```python
from build123d import *

# Parameters (mm, degrees)
BOSS_EXTRUDE1_DEPTH = 12.7
SKETCH2_R           = 3.175000002
CUT_EXTRUDE1_DEPTH  = 2375.892579794


with BuildPart() as part:
    # Sketch1 → Boss-Extrude1 (new body)
    with BuildSketch(Plane(origin=(-0.000661708, -8255.328766721, 681.010699718), x_dir=(-0.9999999999999969, 7.961414168714261e-08, -6.567661367452003e-09), z_dir=(-7.988457756299225e-08, -0.996614682353027, 0.08221420143970737))):
        Polygon((927.932358973, -1893.28840213), (1306.839320092, -1893.28840213), (1432.35206282, -1316.739819062), (802.419616245, -1316.739819062), align=None)
    extrude(amount=BOSS_EXTRUDE1_DEPTH)

    # Sketch2 → Cut-Extrude1 (cut, through all)
    with BuildSketch(Plane(origin=(-0.000661714, -8255.328766721, 681.010699718), x_dir=(0.9999999999999968, -7.961414422751635e-08, 6.5676468617910225e-09), z_dir=(7.988457890219468e-08, 0.9966146823530272, -0.08221420143970452))):
        with Locations(Location((-1284.956595837, -1854.019614904, 0), (0, 0, 270))):
            Circle(SKETCH2_R)
        with Locations(Location((-949.797461581, -1853.938669103, 0), (0, 0, 270))):
            Circle(SKETCH2_R)
        with Locations(Location((-1387.301054815, -1360.701208825, 0), (0, 0, 270))):
            Circle(SKETCH2_R)
        with Locations(Location((-847.47062424, -1360.701208825, 0), (0, 0, 270))):
            Circle(SKETCH2_R)
    extrude(amount=-CUT_EXTRUDE1_DEPTH, mode=Mode.SUBTRACT)


solid = part.part
```
Can you work these out from the model? Positions are in its coordinate system, mm. Give positions to 0.01 mm unless a question says otherwise; leave off trailing zeros. Loops run counter-clockwise (first coordinate to the right, second up) from the corner with the lowest first, then second, coordinate; pieces in that order, holes last. Notation, with made-up numbers: M -5.5,29.25 L 33.5,29.25 A19 cw 33.5,39.25 Z; hole C -5.5,50.5 d6. An arc over 180 degrees is marked long. One line per question, with ' | ' between items. Start each with the question number.
Q1. For pin 1 Ø1.5 at (x, z) = (-1346, 2326) entering from +Y; pin 2 Ø3 at (y, z) = (-8142, 2217.5) entering from -X; pin 3 Ø4 at (x, z) = (-1267, 2114) entering from -Y, each with a flat end and sliding along its axis, tell me the tip position at first contact or that it passes through.
Q2. If I drill on line 1 (Y direction, x = -963.5, z = 2105.5); line 2 (Y direction, x = -1050.5, z = 2347.5), over which ranges is the centre line in solid material (lowest first)? Write a range as from..to.
Q3. If we section it at A-A (x = -987.5): Please give me the cut outline in (y, z), plus the area to 3 significant figures.
Q4. If we section it at B-B (z = 2301): Please give me the cut outline in (x, y), plus the area to 3 significant figures.
Computed:
1) pin 1: stops at y = -8119.57 | pin 2: stops at x = -1383.91 | pin 3: stops at y = -8150.02
2) line 1: y = -8150.56..-8137.82 | line 2: y = -8130.6..-8117.85
3) outline: M -8159.73,1994.34 L -8147.07,1993.29 L -8099.67,2567.89 L -8112.33,2568.93 Z | area: 7,320 mm²
4) outline: M -1365.37,-8134.43 L -869.41,-8134.43 L -869.63,-8121.69 L -1365.14,-8121.69 Z | area: 6,320 mm²
